from build123d import *

# Parameters (mm, degrees)
F0_W     = 60
F0_H     = 60
F1_DEPTH = 30
F2_DEPTH = 30
F3_R     = 20
F4_DEPTH = 10
F6_R     = 15.3845355262
F7_DEPTH = 10
F8_W     = 60
F8_H     = 60
F9_DEPTH = 4


with BuildPart() as f1:
    # F0 (on Top) → F1 (new body)
    with BuildSketch(Plane.XY):
        Rectangle(F0_W, F0_H)
    extrude(amount=F1_DEPTH)

    # F2 (add): a face of the model
    f2_faces = [f1.faces().sort_by_distance(p)[0] for p in [
        (0, 0, 0),
    ]]
    extrude(f2_faces, amount=F2_DEPTH)

    # F3 (on face) → F4 (join)
    with BuildSketch(Plane.XY.offset(30)):
        Circle(F3_R)
    extrude(amount=F4_DEPTH)

    # F6 (on face) → F7 (cut)
    with BuildSketch(Plane.XY.offset(40)):
        Circle(F6_R)
    extrude(amount=-F7_DEPTH, mode=Mode.SUBTRACT)

    # F8 (on face) → F9 (cut)
    with BuildSketch(Plane(origin=(0, 30, 0), x_dir=(-1, 0, 0), z_dir=(0, 1, 0))):
        Rectangle(F8_W, F8_H)
    extrude(amount=F9_DEPTH, mode=Mode.SUBTRACT)


solid = f1.part
Geometry check sheet. Reference: the model listing, model coordinates, mm. A direction names the side the tool comes from. Round coordinates to 2 decimals unless told otherwise and drop trailing zeros. Loops run counter-clockwise (first coordinate to the right, second up) from the corner with the lowest first, then second, coordinate; pieces in that order, holes last.
Item 1: Cross-section at C-C on y = 23. Record the boundary of the cut face in (x, z).
Item 2: Cross-section at A-A on x = 0. Record the boundary of the cut face in (y, z).
Item 3: Access from +Z, -Z, +X, -X, +Y, -Y to the whole of each face (thin tool, end or side, straight path). Record for faces 5 (the cylindrical face through (-4.336, -19.524, 34.93)), 6 (the flat face through (0, 30, 0)).
Item 4: Mould release check, pull along Y, two halves, no side actions. Record for faces 1 (the flat face through (10, -12, 40)), 2 (the flat face through (0, -30, 0)), 3 (the cylindrical face through (-3.335, -15.019, 35.07)), 4 (the flat face through (0, 0, 30)): pulls with the +Y half, pulls with the -Y half, needs draft (parallel to the pull), parting line crosses it, or undercut.
Item 5: Gauge pin test, flat ends, axial feed: pin 1 (4 mm diameter, centred on x = 1.5, y = 3.5, fed in from +Z); pin 2 (4 mm diameter, centred on x = 15.5, z = 32.5, fed in from +Y). Record the tip position at first contact, or that the pin passes through.
Item 6: Thickness scan on line 1 (Y direction, x = 0, z = 36); line 2 (Z direction, x = 25, y = 17); line 3 (Y direction, x = 2.5, z = 32.5). Record the ranges inside material, lowest first.
Answer sheet:
1. outline: (-30, -30) - (30, -30) - (30, 30) - (-30, 30) - close
2. outline: (-30, -30) - (30, -30) - (30, 30) - (20, 30) - (20, 40) - (15.38, 40) - (15.38, 30) - (-15.38, 30) - (-15.38, 40) - (-20, 40) - (-20, 30) - (-30, 30) - close
3. face 5: +Z
3. face 6: +Z, -Z, +X, -X, +Y
4. face 1: needs draft
4. face 2: pulls with the -Y half
4. face 3: undercut
4. face 4: undercut
5. pin 1: stops at z = 30
5. pin 2: stops at y = 14.76
6. line 1: y = -20 to -15.38, 15.38 to 20
6. line 2: z = -30 to 30
6. line 3: y = -19.84 to -15.18, 15.18 to 19.84
